Source: CAD feature listing. Evaluate the final solid. Frame: model axes, mm. A direction names the side the tool comes from. Coordinates: 2 decimals unless noted, no trailing zeros. Order: outer loops, then holes, each group sorted by start corner. A loop starts at its lowest first (then second) coordinate and runs counter-clockwise, first axis right, second up.
Item 1: Section C-C on x = 8. Return the cut outline in (y, z), then the cut area to 3 significant figures.
Item 2: Ray query, line 1 (X direction, y = 60.7, z = 0.6); line 2 (Y direction, x = 2.75, z = 0.9); line 3 (X direction, y = 35.2, z = 0.8). Return the intervals inside material, ascending.
Item 3: Section B-B on y = 22.94. Return the cut outline in (x, z).
Item 4: Section D-D on y = 47. Return the cut outline in (x, z), then the cut area to 3 significant figures.
Item 5: Reachability of faces 1 (the flat face through (6, 49, 1)), 2 (the flat face through (4, 49, 1)), 3 (the flat face through (3, 20.44, 1)) from +Z, -Z, +X, -X, +Y, -Y: full face, straight path, thin tool, end or side. Return the list, or none.
Item 6: Mould query, pull axis X, two halves, no side actions, for faces 4 (the cylindrical face through (13.9, 42.8, 1)), 5 (the cylindrical face through (0.6, 21.01, 0.99)), 6 (the flat face through (5, 12.44, 1)). Classes: released by +X, released by -X, zero draft, split by the parting line, or undercut.
Item 7: Section A-A on x = 2.75. Return the cut outline in (y, z), then the cut area to 3 significant figures.
Item 8: Contact query for flat-ended pins moving along their axis: P1, Ø2.5, axis at x = 13.45, y = 42.2, coming from the -Z side; P2, Ø1, axis at y = 50.5, z = 1, coming from the +X side; P3, Ø1, axis at x = 2.5, z = 1, coming from the -Y side. Output: stop coordinate, or through.
from build123d import *

# Parameters (mm, degrees)
SKETCH1_R           = 0.75
SKETCH1_R_2         = 0.9
SKETCH1_W           = 4.2
SKETCH1_H           = 8
BOSS_EXTRUDE1_DEPTH = 2


with BuildPart() as part:
    # Sketch1 → Boss-Extrude1 (new body)
    with BuildSketch(Plane.XY):
        with BuildLine():
            Line((4, 44.7), (4, 52.7))
            Line((4, 52.7), (2, 52.7))
            ThreePointArc((2, 52.7), (0.585786438, 53.285786438), (0, 54.7))
            Line((0, 54.7), (0, 67.93))
            Line((0, 67.93), (16.2, 67.93))
            Line((16.2, 67.93), (16.2, 54.7))
            ThreePointArc((16.2, 54.7), (15.614213562, 53.285786438), (14.2, 52.7))
            Line((14.2, 52.7), (12.2, 52.7))
            Line((12.2, 52.7), (12.2, 44.7))
            Line((12.2, 44.7), (14.2, 44.7))
            ThreePointArc((14.2, 44.7), (15.614213562, 44.114213562), (16.2, 42.7))
            Line((16.2, 42.7), (16.2, 22.44))
            ThreePointArc((16.2, 22.44), (15.614213562, 21.025786438), (14.2, 20.44))
            Line((14.2, 20.44), (12.2, 20.44))
            Line((12.2, 20.44), (12.2, 12.44))
            Line((12.2, 12.44), (10.2, 12.44))
            Line((10.2, 12.44), (10.2, 20.44))
            Line((10.2, 20.44), (6, 20.44))
            Line((6, 20.44), (6, 12.44))
            Line((6, 12.44), (4, 12.44))
            Line((4, 12.44), (4, 20.44))
            Line((4, 20.44), (2, 20.44))
            ThreePointArc((2, 20.44), (0.585786438, 21.025786438), (0, 22.44))
            Line((0, 22.44), (0, 42.7))
            ThreePointArc((0, 42.7), (0.585786438, 44.114213562), (2, 44.7))
            Line((2, 44.7), (4, 44.7))
        make_face()
        with Locations((2.75, 60.7)):
            Circle(SKETCH1_R, mode=Mode.SUBTRACT)
        with Locations((13.45, 54.7)):
            Circle(SKETCH1_R, mode=Mode.SUBTRACT)
        with Locations((13.45, 42.2)):
            Circle(SKETCH1_R, mode=Mode.SUBTRACT)
        with Locations((13.45, 22.94)):
            Circle(SKETCH1_R_2, mode=Mode.SUBTRACT)
        with Locations((10.2, 29.94)):
            Circle(SKETCH1_R_2, mode=Mode.SUBTRACT)
        with Locations((6, 35.2)):
            Circle(SKETCH1_R, mode=Mode.SUBTRACT)
        with Locations((13.45, 60.7)):
            Circle(SKETCH1_R, mode=Mode.SUBTRACT)
        with Locations((10.2, 35.2)):
            Circle(SKETCH1_R, mode=Mode.SUBTRACT)
        with Locations((6, 29.94)):
            Circle(SKETCH1_R_2, mode=Mode.SUBTRACT)
        with Locations((2.75, 22.94)):
            Circle(SKETCH1_R_2, mode=Mode.SUBTRACT)
        with Locations((2.75, 42.2)):
            Circle(SKETCH1_R, mode=Mode.SUBTRACT)
        with Locations((2.75, 54.7)):
            Circle(SKETCH1_R, mode=Mode.SUBTRACT)
        with Locations((8.1, 48.7)):
            Rectangle(SKETCH1_W, SKETCH1_H, mode=Mode.SUBTRACT)
    extrude(amount=BOSS_EXTRUDE1_DEPTH)


solid = part.part
Answer list:
1. outline: (20.44, 0) - (44.7, 0) - (44.7, 2) - (20.44, 2) - close; (52.7, 0) - (67.93, 0) - (67.93, 2) - (52.7, 2) - close
1. area: 79.0 mm2
2. line 1: x = 0 to 2, 3.5 to 12.7, 14.2 to 16.2
2. line 2: y = 20.44 to 22.04, 23.84 to 41.45, 42.95 to 44.7, 52.7 to 53.95, 55.45 to 59.95, 61.45 to 67.93
2. line 3: x = 0 to 5.25, 6.75 to 9.45, 10.95 to 16.2
3. outline: (0, 0) - (1.85, 0) - (1.85, 2) - (0, 2) - close; (3.65, 0) - (12.55, 0) - (12.55, 2) - (3.65, 2) - close; (14.35, 0) - (16.2, 0) - (16.2, 2) - (14.35, 2) - close
4. outline: (4, 0) - (6, 0) - (6, 2) - (4, 2) - close; (10.2, 0) - (12.2, 0) - (12.2, 2) - (10.2, 2) - close
4. area: 8.00 mm2
5. face 1: +Z, -Z
5. face 2: +Z, -Z, -X
5. face 3: +Z, -Z, -X, -Y
6. face 4: undercut
6. face 5: released by -X
6. face 6: zero draft
7. outline: (20.44, 0) - (22.04, 0) - (22.04, 2) - (20.44, 2) - close; (23.84, 0) - (41.45, 0) - (41.45, 2) - (23.84, 2) - close; (42.95, 0) - (44.7, 0) - (44.7, 2) - (42.95, 2) - close; (52.7, 0) - (53.95, 0) - (53.95, 2) - (52.7, 2) - close; (55.45, 0) - (59.95, 0) - (59.95, 2) - (55.45, 2) - close; (61.45, 0) - (67.93, 0) - (67.93, 2) - (61.45, 2) - close
7. area: 66.4 mm2
8. P1: stops at z = 0
8. P2: stops at x = 12.2
8. P3: stops at y = 20.44
